Source: CAD feature listing. Evaluate the final solid. Frame: model axes, mm. Face numbers are marked on the shaded views. A direction names the side the tool comes from. Coordinates: 2 decimals unless noted, no trailing zeros. Loops run counter-clockwise (first coordinate to the right, second up) from the corner with the lowest first, then second, coordinate; pieces in that order, holes last. Notation, with made-up numbers: (78.25, 55) - (120.25, 55) arc R14 ccw to (120.25, 67) - close; hole circle Ø3 at (46, 14.25). An arc over 180 degrees is marked (long way). Use one line per item in the form item = value. Start each with the question number.
from build123d import *

# Parameters (mm, degrees)
F0_R     = 1.5
F0_R_2   = 2.5
F1_DEPTH = 5
F3_W     = 5.8
F3_H     = 5.2
F4_DEPTH = 4.5


with BuildPart() as f1:
    # F0 (on Front) → F1 (new body)
    with BuildSketch(Plane.XZ):
        Polygon((34.4082845706, -12.5), (34.4082845706, 12.5), (14.4082845706, 12.5), (-28.5917154294, 12.5), (-28.5917154294, -2.5), (14.4082845706, -2.5), (14.4082845706, -12.5), align=None)
        with Locations((-23.0917154294, 5)):
            Circle(F0_R, mode=Mode.SUBTRACT)
        with Locations((-13.5917154294, 5)):
            Circle(F0_R, mode=Mode.SUBTRACT)
        with Locations((24.4082845706, 0)):
            Circle(F0_R_2, mode=Mode.SUBTRACT)
    extrude(amount=F1_DEPTH)

    # F3 (on offset) → F4 (join)
    with BuildSketch(Plane(origin=(0, 0, 0), x_dir=(-1, 0, 0), z_dir=(0, 1, 0))):
        with Locations((-24.4082845706, 10.0041090116)):
            Rectangle(F3_W, F3_H)
        with Locations((-24.4082845706, -10.0041090116)):
            Rectangle(F3_W, F3_H)
    extrude(amount=F4_DEPTH)


solid = f1.part
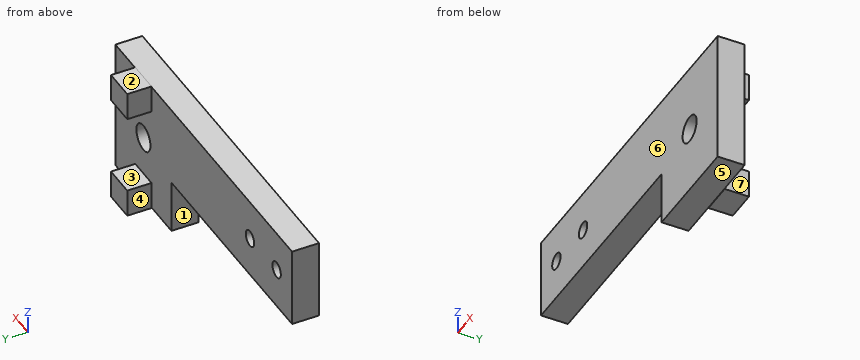
(1) Cut plane B-B, the plane y = 3.5. Output: boundary loops of the cut face in (x, z).
(2) Cut plane D-D, the plane y = -2.25. Output: boundary loops of the cut face in (x, z).
(3) Cut plane C-C, the plane z = 0. Output: boundary loops of the cut face in (x, y), plus the area to 3 significant figures.
(4) Material intervals for line 1 (Z direction, x = 8.5, y = -2); line 2 (Z direction, x = 29, y = -3.5); line 3 (Y direction, x = 24.5, z = 6.5), sorted ascending.
(5) Cut plane A-A, the plane z = 5. Output: boundary loops of the cut face in (x, y).
(6) Contact query for flat-ended pins moving along their axis: pin 1 (12.5 mm diameter, centred on x = -11, z = -4.5, fed in from +Y); pin 2 (1.3 mm diameter, centred on y = 1.5, z = -10, fed in from -X); pin 3 (6.5 mm diameter, centred on x = 24.41, z = 0, fed in from -Y); pin 4 (2.5 mm diameter, centred on x = 27.5, y = -3.5, fed in from -Z). Output: stop coordinate, or through.
(7) Mould query, pull axis Y, two halves, no side actions, for the marked faces 6 and 7. Classes: +Y half, -Y half, draft (parallel to the pull), parting line (faces both ways), or undercut.
(8) Access query for the marked faces 1, 2, 3, 4 and 5. Directions: +Z, -Z, +X, -X, +Y, -Y. A direction counts if a zero-diameter tool reaches every point of the face in a straight line with its end or side. Return the directions, or none.
Recorded:
q1.outline = (21.51, -12.6) - (27.31, -12.6) - (27.31, -7.4) - (21.51, -7.4) - close; (21.51, 7.4) - (27.31, 7.4) - (27.31, 12.6) - (21.51, 12.6) - close
q2.outline = (-28.59, -2.5) - (14.41, -2.5) - (14.41, -12.5) - (34.41, -12.5) - (34.41, 12.5) - (-28.59, 12.5) - close; hole circle Ø3 at (-23.09, 5); hole circle Ø3 at (-13.59, 5); hole circle Ø5 at (24.41, 0)
q3.outline = (-28.59, -5) - (21.91, -5) - (21.91, 0) - (-28.59, 0) - close; (26.91, -5) - (34.41, -5) - (34.41, 0) - (26.91, 0) - close
q3.area = 290 mm²
q4.line_1 = -2.5 to 12.5
q4.line_2 = -12.5 to 12.5
q4.line_3 = -5 to 0
q5.outline = (-28.59, -5) - (-24.59, -5) - (-24.59, 0) - (-28.59, 0) - close; (-21.59, -5) - (-15.09, -5) - (-15.09, 0) - (-21.59, 0) - close; (-12.09, -5) - (34.41, -5) - (34.41, 0) - (-12.09, 0) - close
q6.pin_1 = 0
q6.pin_2 = 21.51
q6.pin_3 = -5
q6.pin_4 = -12.5
q7.face_6 = -Y half
q7.face_7 = draft
q8.face_1 = -Z, -X, +Y, -Y
q8.face_2 = +Z, +X, -X, +Y, -Y
q8.face_3 = +X, -X, +Y
q8.face_4 = +Z, -Z, -X, +Y
q8.face_5 = -Z, +X, -X, -Y
